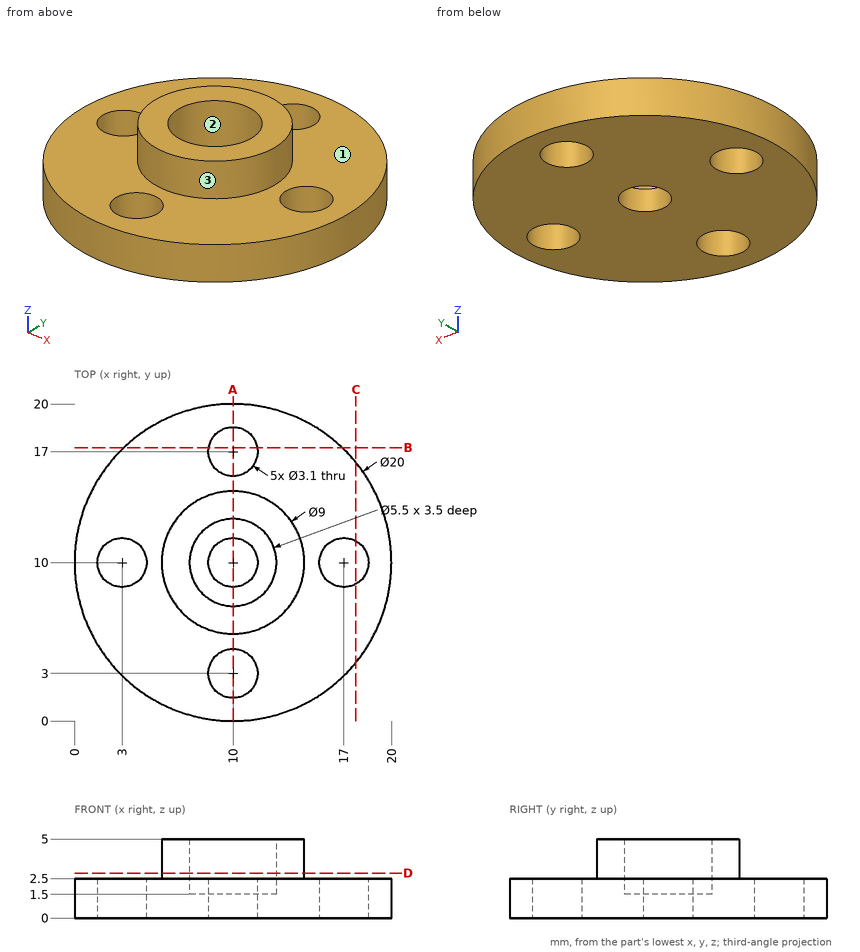
The figure shows three views and two pictorial views of one solid part (mm, origin at its lowest corner). Answer the questions. Coordinates: 2 decimals unless noted, no trailing zeros. Order: outer loops, then holes, each group sorted by start corner. A loop starts at its lowest first (then second) coordinate and runs counter-clockwise, first axis right, second up. Notation, with made-up numbers: (77.25, -22.75) - (103.25, -22.75) arc R22 ccw to (103.25, 16.25) - close; hole circle Ø5 at (39.25, 28.25). An arc over 180 degrees is marked (long way). Answer as a JSON object with one key per item and string values.
1. Find section B-B on y = 17.25. Determine the outline of the cut face in (x, z), plus the area to 3 significant figures.
Output values:
{"outline": "(3.11, 0) - (8.47, 0) - (8.47, 2.5) - (3.11, 2.5) - close; (11.53, 0) - (16.89, 0) - (16.89, 2.5) - (11.53, 2.5) - close", "area": "26.8 mm²"}
2. Find section A-A on x = 10. Determine the outline of the cut face in (y, z), plus the area to 3 significant figures.
Output values:
{"outline": "(0, 0) - (1.45, 0) - (1.45, 2.5) - (0, 2.5) - close; (4.55, 0) - (8.45, 0) - (8.45, 1.5) - (7.25, 1.5) - (7.25, 5) - (5.5, 5) - (5.5, 2.5) - (4.55, 2.5) - close; (11.55, 0) - (15.45, 0) - (15.45, 2.5) - (14.5, 2.5) - (14.5, 5) - (12.75, 5) - (12.75, 1.5) - (11.55, 1.5) - close; (18.55, 0) - (20, 0) - (20, 2.5) - (18.55, 2.5) - close", "area": "33.1 mm²"}
3. Find section D-D on z = 2.85. Determine the outline of the cut face in (x, y).
Output values:
{"outline": "circle Ø9 at (10, 10); hole circle Ø5.5 at (10, 10)"}
4. Find section C-C on x = 17.75. Determine the outline of the cut face in (y, z), plus the area to 3 significant figures.
Output values:
{"outline": "(3.68, 0) - (8.64, 0) - (8.64, 2.5) - (3.68, 2.5) - close; (11.36, 0) - (16.32, 0) - (16.32, 2.5) - (11.36, 2.5) - close", "area": "24.8 mm²"}
5. The mould has two halves that part along X. Classify the marked faces 1, 2 and 3: +X half, -X half, draft (parallel to the pull), parting line (faces both ways), or undercut.
Output values:
{"face 1": "draft", "face 2": "undercut", "face 3": "parting line"}
6. Consider line 1 (Y direction, x = 10, z = 0.85); line 2 (Y direction, x = 10, z = 3.9); line 3 (Z direction, x = 1, y = 14). Determine where each line is inside the solid, lowest interval first.
Output values:
{"line 1": "y = 0 to 1.45, 4.55 to 8.45, 11.55 to 15.45, 18.55 to 20", "line 2": "y = 5.5 to 7.25, 12.75 to 14.5", "line 3": "z = 0 to 2.5"}
7. Each of these flat-tipped pins is pushed along its axis until it touches: P1, Ø3.5, axis at x = 3, y = 10, coming from the +Z side; P2, Ø3, axis at y = 2, z = 2.5, coming from the -X side; P3, Ø1, axis at x = 12, z = 3.5, coming from the +Y side. Where does it stop, or does it pass through?
Output values:
{"P1": "stops at z = 2.5", "P2": "stops at x = 2.4", "P3": "stops at y = 14.24"}
